```python
from build123d import *

# Parameters (mm, degrees)
PAD_DEPTH = 3.175


with BuildPart() as part:
    # Sketch → Pad (new body)
    with BuildSketch(Plane.XZ):
        with BuildLine():
            ThreePointArc((-17.018, 2.487326), (-2.996285, 8.327774), (7.609137, 19.201797))
            Line((7.609137, 19.201797), (8.633146, 19.201797))
            Line((8.633146, 19.201797), (9.610686, 16.733412))
            Line((9.610686, 16.733412), (10.867529, 13.800783))
            Line((10.867529, 13.800783), (11.991159, 9.834628))
            ThreePointArc((14.591504, 8.819976), (13.334049, 9.436779), (11.991159, 9.834628))
            ThreePointArc((16.220824, 4.677015), (16.131692, 7.033827), (14.591504, 8.819976))
            ThreePointArc((14.5915, 1.790975), (15.512541, 3.173938), (16.220824, 4.677015))
            Line((15.24005, 0.007885), (14.5915, 1.790975))
            Line((16.310692, -3.716085), (15.24005, 0.007885))
            Line((17.381336, -7.533156), (16.310692, -3.716085))
            Line((16.453487, -8.310298), (17.381336, -7.533156))
            ThreePointArc((16.453487, -8.310298), (8.209274, -5.944046), (-0.364355, -5.701006))
            Line((-0.734469, -6.577293), (-0.364355, -5.701006))
            Line((-0.958348, -8.024061), (-0.734469, -6.577293))
            Line((-1.152321, -10.465385), (-0.958348, -8.024061))
            Line((-0.608809, -13.055986), (-1.152321, -10.465385))
            Line((0.885784, -17.303194), (-0.608809, -13.055986))
            Line((0.602916, -17.861423), (0.885784, -17.303194))
            Line((-2.274875, -19.050779), (0.602916, -17.861423))
            Line((-3.953837, -18.944079), (-2.274875, -19.050779))
            Line((-10.490349, -8.764157), (-3.953837, -18.944079))
            Line((-11.290691, -8.230595), (-10.490349, -8.764157))
            Line((-12.586489, -8.916603), (-11.290691, -8.230595))
            Line((-13.424941, -8.726046), (-12.586489, -8.916603))
            Line((-15.254302, -5.982009), (-13.424941, -8.726046))
            Line((-15.787862, -5.867674), (-15.254302, -5.982009))
            Line((-16.969324, -5.334111), (-15.787862, -5.867674))
            Line((-17.693443, -4.190763), (-16.969324, -5.334111))
            Line((-17.502886, -2.818745), (-17.693443, -4.190763))
            Line((-16.550095, -1.561061), (-17.502886, -2.818745))
            Line((-17.018, 2.487326), (-16.550095, -1.561061))
        make_face()
    extrude(amount=PAD_DEPTH)


solid = part.part
```
Here's how the part is built. I have some questions about the finished solid (model axes, mm). A direction names the side the tool comes from. Round coordinates to 2 decimals unless told otherwise and drop trailing zeros. Order: outer loops, then holes, each group sorted by start corner. A loop starts at its lowest first (then second) coordinate and runs counter-clockwise, first axis right, second up. Notation, with made-up numbers: (57, 0) -> (81, 0) arc R28 ccw to (81, 27) -> close; hole circle Ø9 at (-25, 84.25). An arc over 180 degrees is marked (long way). Use a Markdown table: item, result. Add a question column.
(1) For faces 1 (the face through (-16.787, -1.565, 0.491)), 2 (the face through (14.92, -1.57, 0.89)), 3 (the face through (10.23, -1.57, 15.29)), which set-ups out of +Z, -Z, +X, -X, +Y, -Y let a thin tool reach every point of the face, with its end or its side?
(2) I need wall thicknesses on line 1 along Z through (x, y) = (8.5, -2.05); line 2 along X through (y, z) = (-0.1, -8); line 3 along X through (y, z) = (-0.85, -9). Which ranges of each line are inside material? Lowest first, please.
(3) If we mould it in two halves opening along Z, with no side actions, what happens to faces 4 (the face through (15.783, -1.565, -1.88)), 5 (the face through (-7.27, -1.57, -13.78)), 6 (the face through (-3.17, -1.57, 8.21))? For each: released by +Z, released by -Z, zero draft, split by the parting line, or undercut.
(4) Suppose I cut it at C-C, the plane x = 13.5. Please give me the cut outline in (y, z) (3 decimals), and give its area (3 significant figures).
(5) Suppose I cut it at B-B, the plane z = -2. Please give me the cut outline in (x, y) (3 decimals), and give its area (3 significant figures).
Verdict:
| question | item | result |
|---|---|---|
| 1 | face 1 | -X, +Y, -Y |
| 1 | face 2 | +X, +Y, -Y |
| 1 | face 3 | +Z, +X, +Y, -Y |
| 2 | line 1 | -5.99 to 19.2 |
| 2 | line 2 | -13.91 to -0.95, 15.71 to 16.82 |
| 2 | line 3 | -10.34 to -1.04 |
| 3 | face 4 | undercut |
| 3 | face 5 | released by -Z |
| 3 | face 6 | released by +Z |
| 4 | outline | (-3.175, -7.202) -> (0, -7.202) -> (0, 9.37) -> (-3.175, 9.37) -> close |
| 4 | area | 52.6 mm2 |
| 5 | outline | (-16.883, -3.175) -> (15.817, -3.175) -> (15.817, 0) -> (-16.883, 0) -> close |
| 5 | area | 104 mm2 |
